For this review, take the finished solid that the model builds, in its own axes (mm). A direction names the side the tool comes from. Coordinates: 2 decimals unless noted, no trailing zeros. Loops run counter-clockwise (first coordinate to the right, second up) from the corner with the lowest first, then second, coordinate; pieces in that order, holes last. Notation, with made-up numbers: (-33.75, -40) - (-29.75, -40) arc R17 cw to (-29.75, -32) - close; hole circle Ø8 at (-6, 3.5). An arc over 180 degrees is marked (long way). Answer as a JSON object with one key per item and string values. Group by question number.
Item 1: To check wall thickness, follow line 1 (Y direction, x = 136, z = 35.65); line 2 (X direction, y = -21.5, z = 27.6); line 3 (Y direction, x = 136, z = 28.2). State the ranges of each line that lie inside material, in increasing order.
Item 2: We need section C-C (z = 33.5). Give the boundary of the cut face in (x, y).
Item 3: Mouldability with a two-part tool opening along Y and no side actions: class faces 1 (the flat face through (136, -22, 30)), 2 (the cylindrical face through (140.619, -23.415, 33.24)), 3 (the flat face through (135, -19, 35.5)) as released by +Y, released by -Y, zero draft, split by the parting line, or undercut.
Item 4: We need section B-B (x = 136). Give the boundary of the cut face in (y, z).
Item 5: We need section A-A (y = -21.5). Give the boundary of the cut face in (x, z).
Item 6: Clearance check with flat-ended pins moving along their axes: pin 1 (2 mm diameter, centred on y = -24.5, z = 34.5, fed in from -X); pin 2 (2.5 mm diameter, centred on x = 136, y = -21.5, fed in from -Z); pin 3 (2 mm diameter, centred on x = 135, z = 27.5, fed in from +Y). State where each tip first meets the part, or that it passes through.
Item 7: We need section D-D (z = 29.5). Give the boundary of the cut face in (x, y).
Item 8: Tool access review of faces 4 (the flat face through (137, -20, 26)), 5 (the flat face through (137, -19, 32.5)), 6 (the flat face through (136, -21, 35.5)): name each direction out of +Z, -Z, +X, -X, +Y, -Y from which nothing blocks a thin tool from reaching the whole face with its end or side.
from build123d import *

# Parameters (mm, degrees)
SKETCH046_R     = 2.5
PAD023_DEPTH    = 2.5
SKETCH047_R     = 5
PAD024_DEPTH    = 3
FILLET003_R     = 1.5
SKETCH049_R     = 2.5
PAD025_DEPTH    = 4
SKETCH050_R     = 1.5
POCKET026_DEPTH = 4
SKETCH092_R     = 2.5
SKETCH092_R_2   = 2
PAD058_DEPTH    = 0.2


with BuildPart() as part:
    # Sketch046 → Pad023 (new body)
    with BuildSketch(Plane(origin=(0, 0, 30), x_dir=(1, 0, 0), z_dir=(0, 0, -1))):
        with Locations((101, 55)):
            Circle(SKETCH046_R)
    extrude(amount=-PAD023_DEPTH)

    # Sketch047 (on Face3 of Pad023) → Pad024 (join)
    with BuildSketch(Plane.XY.offset(32.5)):
        with Locations((101, -55)):
            Circle(SKETCH047_R)
    extrude(amount=PAD024_DEPTH)

    # Fillet003
    fillet003_edges = [part.edges().sort_by_distance(p)[0] for p in [
        (96, -55, 35.5),
    ]]
    fillet(fillet003_edges, radius=FILLET003_R)

    # Sketch049 → Pad025 (join)
    with BuildSketch(Plane(origin=(0, 0, 30), x_dir=(1, 0, 0), z_dir=(0, 0, -1))):
        with Locations((101, 55)):
            Circle(SKETCH049_R)
    extrude(amount=PAD025_DEPTH)

    # Sketch050 (on Face17 of Pad025) → Pocket026 (cut)
    with BuildSketch(Plane(origin=(0, 0, 26), x_dir=(1, 0, 0), z_dir=(0, 0, -1))):
        with Locations((101, 55)):
            Circle(SKETCH050_R)
    extrude(amount=-POCKET026_DEPTH, mode=Mode.SUBTRACT)


with BuildPart() as part_1:
    # Body002 placement: moved
    add(part.part.moved(Location((75, 0, 0))))

    # Sketch092 (on Face4 of Clone006) → Pad058 (new body)
    with BuildSketch(Plane(origin=(75, 0, 35.5), x_dir=(1, 0, 0), z_dir=(0, 0, 1))):
        with Locations((101, -55)):
            Circle(SKETCH092_R)
        with Locations((101, -55)):
            Circle(SKETCH092_R_2, mode=Mode.SUBTRACT)
    extrude(amount=PAD058_DEPTH)


with BuildPart() as part_2:
    # Body015 placement: moved
    add(part_1.part.moved(Location((-40, 33.5, 0))))


solid = part_2.part
Check sheet entries:
{
 "1": {"line 1": "y = -24 to -23.5, -19.5 to -19", "line 2": "x = 133.5 to 134.5, 137.5 to 138.5", "line 3": "y = -24 to -23, -20 to -19"},
 "2": {"outline": "circle Ø10 at (136, -21.5)"},
 "3": {"face 1": "undercut", "face 2": "split by the parting line", "face 3": "zero draft"},
 "4": {"outline": "(-26.5, 32.5) - (-24, 32.5) - (-24, 26) - (-23, 26) - (-23, 30) - (-20, 30) - (-20, 26) - (-19, 26) - (-19, 32.5) - (-16.5, 32.5) - (-16.5, 34) arc R1.5 ccw to (-18, 35.5) - (-19, 35.5) - (-19, 35.7) - (-19.5, 35.7) - (-19.5, 35.5) - (-23.5, 35.5) - (-23.5, 35.7) - (-24, 35.7) - (-24, 35.5) - (-25, 35.5) arc R1.5 ccw to (-26.5, 34) - close"},
 "5": {"outline": "(131, 32.5) - (133.5, 32.5) - (133.5, 26) - (134.5, 26) - (134.5, 30) - (137.5, 30) - (137.5, 26) - (138.5, 26) - (138.5, 32.5) - (141, 32.5) - (141, 34) arc R1.5 ccw to (139.5, 35.5) - (138.5, 35.5) - (138.5, 35.7) - (138, 35.7) - (138, 35.5) - (134, 35.5) - (134, 35.7) - (133.5, 35.7) - (133.5, 35.5) - (132.5, 35.5) arc R1.5 ccw to (131, 34) - close"},
 "6": {"pin 1": "stops at x = 131.45", "pin 2": "stops at z = 30", "pin 3": "stops at y = -19"},
 "7": {"outline": "circle Ø5 at (136, -21.5); hole circle Ø3 at (136, -21.5)"},
 "8": {"face 4": "-Z, +X, -X, +Y, -Y", "face 5": "-Z", "face 6": "+Z"}
}
